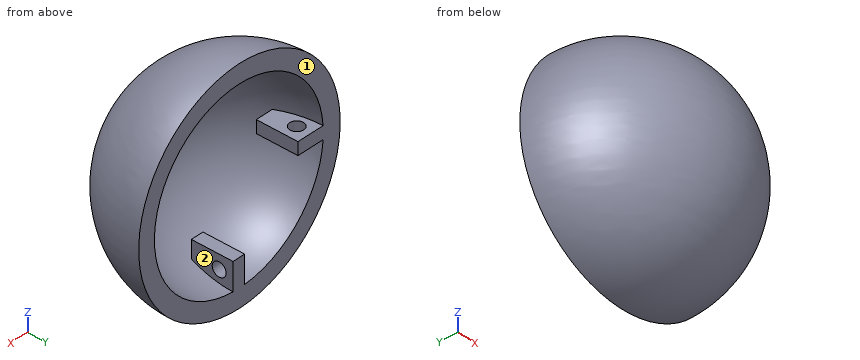
from build123d import *

# Parameters (mm, degrees)
REVOLVE1_ANGLE      = 180
SKETCH3_W           = 1.371722334
SKETCH3_H           = 4
SKETCH3_W_2         = 4
SKETCH3_H_2         = 1.371722334
BOSS_EXTRUDE1_DEPTH = 4.5
CUT_EXTRUDE1_REACH  = 23.148
SKETCH4_R           = 0.75
CUT_EXTRUDE2_REACH  = 23.148
SKETCH5_R           = 0.75


with BuildPart() as part:
    # Sketch1 → Revolve1 (revolve)
    with BuildSketch(Plane(origin=(0, 0, 0), x_dir=(1, 0, 0), z_dir=(0, 1, 0))):
        with BuildLine():
            Line((-0.14015916, 11.999181447), (0, -12))
            ThreePointArc((0, -12), (-11.99979536, -0.070080775), (-0.14015916, 11.999181447))
        make_face()
    revolve(axis=Axis((-0.14015916, 0, -11.999181447), (0.005840064605885622, 0, 0.9999829466772917)), revolution_arc=REVOLVE1_ANGLE)

    # Sketch2 → Cut-Revolve1 (revolve, cut)
    with BuildSketch(Plane(origin=(0, 0, 0), x_dir=(1, 0, 0), z_dir=(0, 1, 0))):
        with BuildLine():
            Line((0, -10), (0, 10))
            ThreePointArc((0, 10), (-10, 0), (0, -10))
        make_face()
    revolve(axis=Axis((0, 0, 10), (0, 0, -1)), mode=Mode.SUBTRACT)

    # Sketch3 → Boss-Extrude1 (add)
    with BuildSketch(Plane(origin=(0, 0, 0), x_dir=(1, 0, 0), z_dir=(0, 1, 0))):
        with Locations((0, 8.99979536)):
            Rectangle(SKETCH3_W, SKETCH3_H)
        with Locations((-8.99979536, 0)):
            Rectangle(SKETCH3_W_2, SKETCH3_H_2)
    extrude(amount=-BOSS_EXTRUDE1_DEPTH)

    # Sketch4 → Cut-Extrude1 (cut, up to next)
    with BuildSketch(Plane(origin=(0, 0, -0.685861167), x_dir=(-1, 0, 0), z_dir=(0, 0, -1)), mode=Mode.PRIVATE) as cut_extrude1_sk1:
        with Locations((8.49979536, -1.5)):
            Circle(SKETCH4_R)
    cut_extrude1_tool1 = extrude(cut_extrude1_sk1.sketch, amount=-CUT_EXTRUDE1_REACH, mode=Mode.PRIVATE) & part.part
    add(cut_extrude1_tool1.solids().sort_by_distance((-8.499795, -1.5, -0.685861))[0], mode=Mode.SUBTRACT)

    # Sketch5 → Cut-Extrude2 (cut, up to next)
    with BuildSketch(Plane(origin=(0.685861167, 0, 0), x_dir=(0, 0, -1), z_dir=(1, 0, 0)), mode=Mode.PRIVATE) as cut_extrude2_sk1:
        with Locations((8.49979536, -1.5)):
            Circle(SKETCH5_R)
    cut_extrude2_tool1 = extrude(cut_extrude2_sk1.sketch, amount=-CUT_EXTRUDE2_REACH, mode=Mode.PRIVATE) & part.part
    add(cut_extrude2_tool1.solids().sort_by_distance((0.685861, -1.5, -8.499795))[0], mode=Mode.SUBTRACT)


solid = part.part
The model under review builds one solid part; all positions refer to its coordinate system, in mm. Face numbers are marked on the shaded views. Round coordinates to 2 decimals unless told otherwise and drop trailing zeros. Return JSON: item names as keys, results as strings.
1. Take a section at A-A (y = -1.5). State how many separate pieces and enclosed holes the cut face has, then the cut area to 3 significant figures.
Answer block:
{"separate pieces": "3", "enclosed holes": "1", "area": "139 mm²"}
2. Insertion check: P1, Ø1.5, axis at x = -0.5, y = -1.5, coming from the +Z side; P2, Ø1.5, axis at y = -3, z = -8.5, coming from the -X side; P3, Ø1.7, axis at x = -8.5, y = -1.5, coming from the -Z side. Each pin has a flat end and moves straight along its axis. Give the tip position at first contact, or say it passes through.
Answer block:
{"P1": "stops at z = 11.97", "P2": "stops at x = -8.7", "P3": "stops at z = -9.13"}
3. The part is to be moulded in two halves that separate along X. For the marked faces 1 and 2, say which applies: +X half, -X half, draft (parallel to the pull), parting line (faces both ways), or undercut.
Answer block:
{"face 1": "draft", "face 2": "undercut"}
4. For L1, parallel to X at y = -7.75, z = 0.25; L2, parallel to X at y = -4.25, z = 3; L3, parallel to Z at x = -7.75, y = -4, list the stretches that pass through material, from the lowest coordinate up. Write a range as [from, to].
Answer block:
{"L1": "x = [-9.14, -6.31], [6.31, 9]", "L2": "x = [-10.81, -8.54], [8.54, 10.67]", "L3": "z = [-8.23, -4.89], [-0.69, 0.69], [4.89, 8.23]"}
